The listing builds one solid part. Answer for the finished solid, in the listing's coordinates (mm). Round coordinates to 2 decimals unless told otherwise and drop trailing zeros. Loops run counter-clockwise (first coordinate to the right, second up) from the corner with the lowest first, then second, coordinate; pieces in that order, holes last. Notation, with made-up numbers: M 32.25,80 L 71.25,80 A29 cw 71.25,101 Z; hole C 54.25,-40 d11. An arc over 180 degrees is marked long. Answer as a JSON object with one key per item and string values.
```python
from build123d import *

# Parameters (mm, degrees)
SKETCH1_W           = 301.625
SKETCH1_H           = 301.625
BOSS_EXTRUDE1_DEPTH = 11.90625
CHAMFER1_SIZE       = 212.725


with BuildPart() as part:
    # Sketch1 → Boss-Extrude1 (new body)
    with BuildSketch(Plane.XY):
        Rectangle(SKETCH1_W, SKETCH1_H)
    extrude(amount=BOSS_EXTRUDE1_DEPTH)

    # Chamfer1
    chamfer1_edges = [part.edges().sort_by_distance(p)[0] for p in [
        (150.8125, -150.8125, 5.953125),
    ]]
    chamfer(chamfer1_edges, length=CHAMFER1_SIZE)


solid = part.part
```
Item 1: Straight lines are drawn through the part: line 1 (X direction, y = -71.5, z = 11.25); line 2 (X direction, y = -31, z = 7.5); line 3 (Y direction, x = 6, z = 7). For each, find the intervals that lie inside material, in ascending order.
Values follow:
{"line 1": "-150.81 to 17.4", "line 2": "-150.81 to 57.9", "line 3": "-82.9 to 150.81"}
Item 2: The part is cut by section C-C (y = -7). Give the vertices of the cut face in (x, z).
Values follow:
{"outline": "M -150.81,0 L 81.9,0 L 81.9,11.91 L -150.81,11.91 Z"}
Item 3: The part is cut by section B-B (x = 11.5). Give the vertices of the cut face in (y, z), then the cut area to 3 significant figures.
Values follow:
{"outline": "M -77.4,0 L 150.81,0 L 150.81,11.91 L -77.4,11.91 Z", "area": "2,720 mm^2"}
Item 4: Flat-ended cylindrical pins translate along their axes: P1, Ø1, axis at y = 55.5, z = 1.5, coming from the +X side; P2, Ø3, axis at y = -81.5, z = 2, coming from the +X side; P3, Ø5, axis at x = -15, z = 7, coming from the -Y side. Find the tip coordinate at first contact, or state that the pin passes through.
Values follow:
{"P1": "x = 144.9", "P2": "x = 8.9", "P3": "y = -106.4"}
Item 5: The part is cut by section A-A (z = 3). Give the vertices of the cut face in (x, y), then the cut area to 3 significant figures.
Values follow:
{"outline": "M -150.81,-150.81 L -61.91,-150.81 L 150.81,61.91 L 150.81,150.81 L -150.81,150.81 Z", "area": "68,400 mm^2"}
